Verification items for this drawing (mm, ordinates from the low corner). Coordinates: 2 decimals unless noted, no trailing zeros. Order: outer loops, then holes, each group sorted by start corner. A loop starts at its lowest first (then second) coordinate and runs counter-clockwise, first axis right, second up. Notation, with made-up numbers: (-13.75, -33) -> (24.25, -33) arc R14 ccw to (24.25, -16) -> close; hole circle Ø1 at (-29.75, 47.5). An arc over 180 degrees is marked (long way). Put each result on its own line as item: value. Start each with the question number.
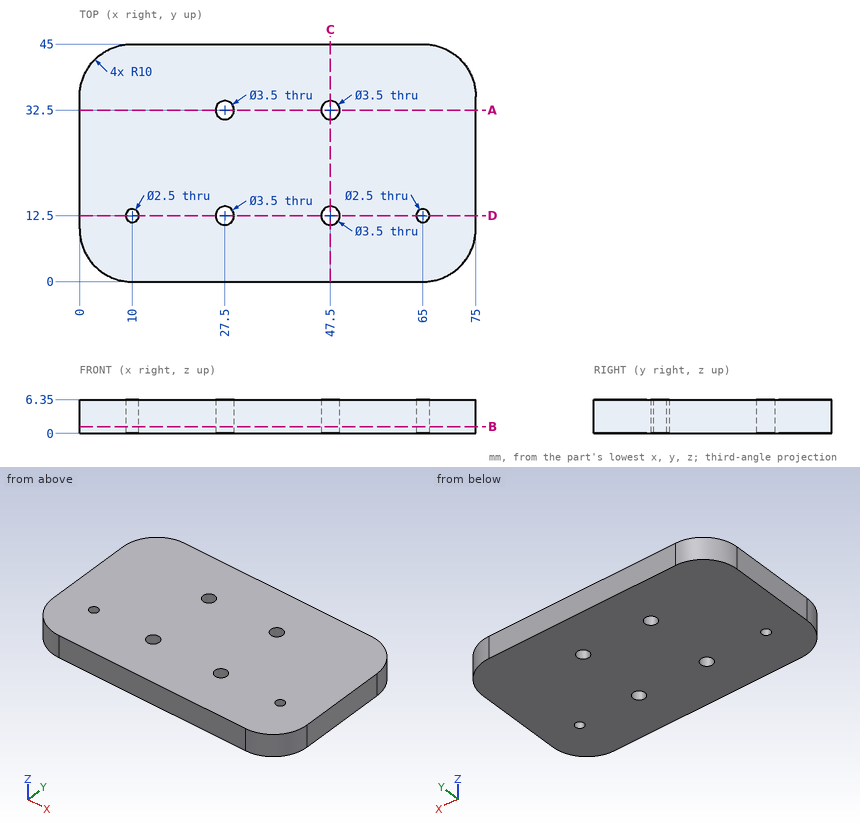
1) Sectioned sample at B-B (z = 1.25). Record the boundary of the cut face in (x, y), plus the area to 3 significant figures.
2) Scan lines: line 1 along Y through (x, z) = (47.5, 4.5); line 2 along X through (y, z) = (12, 5); line 3 along X through (y, z) = (11.5, 2.75). Record each from-to range of solid material in increasing order. Write a range as [from, to].
3) Sectioned sample at C-C (x = 47.5). Record the boundary of the cut face in (y, z), plus the area to 3 significant figures.
4) Sectioned sample at A-A (y = 32.5). Record the boundary of the cut face in (x, z), plus the area to 3 significant figures.
5) Sectioned sample at D-D (y = 12.5). Record the boundary of the cut face in (x, z), plus the area to 3 significant figures.
6) Gauge pin test, flat end, axial feed: pin 1 (2 mm diameter, centred on x = 10, y = 12.5, fed in from -Z). Record the tip position at first contact, or that the pin passes through.
Entries:
1. outline: (0, 10) arc R10 ccw to (10, 0) -> (65, 0) arc R10 ccw to (75, 10) -> (75, 35) arc R10 ccw to (65, 45) -> (10, 45) arc R10 ccw to (0, 35) -> close; hole circle Ø2.5 at (10, 12.5); hole circle Ø3.5 at (27.5, 12.5); hole circle Ø3.5 at (27.5, 32.5); hole circle Ø3.5 at (47.5, 12.5); hole circle Ø3.5 at (47.5, 32.5); hole circle Ø2.5 at (65, 12.5)
1. area: 3,240 mm2
2. line 1: y = [0, 10.75], [14.25, 30.75], [34.25, 45]
2. line 2: x = [0, 8.85], [11.15, 25.82], [29.18, 45.82], [49.18, 63.85], [66.15, 75]
2. line 3: x = [0, 9.25], [10.75, 26.06], [28.94, 46.06], [48.94, 64.25], [65.75, 75]
3. outline: (0, 0) -> (10.75, 0) -> (10.75, 6.35) -> (0, 6.35) -> close; (14.25, 0) -> (30.75, 0) -> (30.75, 6.35) -> (14.25, 6.35) -> close; (34.25, 0) -> (45, 0) -> (45, 6.35) -> (34.25, 6.35) -> close
3. area: 241 mm2
4. outline: (0, 0) -> (25.75, 0) -> (25.75, 6.35) -> (0, 6.35) -> close; (29.25, 0) -> (45.75, 0) -> (45.75, 6.35) -> (29.25, 6.35) -> close; (49.25, 0) -> (75, 0) -> (75, 6.35) -> (49.25, 6.35) -> close
4. area: 432 mm2
5. outline: (0, 0) -> (8.75, 0) -> (8.75, 6.35) -> (0, 6.35) -> close; (11.25, 0) -> (25.75, 0) -> (25.75, 6.35) -> (11.25, 6.35) -> close; (29.25, 0) -> (45.75, 0) -> (45.75, 6.35) -> (29.25, 6.35) -> close; (49.25, 0) -> (63.75, 0) -> (63.75, 6.35) -> (49.25, 6.35) -> close; (66.25, 0) -> (75, 0) -> (75, 6.35) -> (66.25, 6.35) -> close
5. area: 400 mm2
6. pin 1: passes through
